from build123d import *

# Parameters (mm, degrees)
SKETCH1_R           = 13.25
SKETCH1_R_2         = 11.25
BOSS_EXTRUDE1_DEPTH = 7
SKETCH2_R           = 20
BOSS_EXTRUDE2_DEPTH = 2
FILLET1_R           = 6
SKETCH3_R           = 11.25
CUT_EXTRUDE1_DEPTH  = 2
FILLET2_R           = 1


with BuildPart() as part:
    # Sketch1 → Boss-Extrude1 (new body)
    with BuildSketch(Plane.XY):
        Circle(SKETCH1_R)
        Circle(SKETCH1_R_2, mode=Mode.SUBTRACT)
    extrude(amount=BOSS_EXTRUDE1_DEPTH)

    # Sketch2 → Boss-Extrude2 (add)
    with BuildSketch(Plane.XY.offset(7)):
        Circle(SKETCH2_R)
    extrude(amount=-BOSS_EXTRUDE2_DEPTH)

    # Fillet1
    # the kernel refuses this fillet: 6 mm, written as the material it adds along each edge
    with BuildSketch(Plane(origin=(0, 0, 5), x_dir=(1, 0, 0), z_dir=(0, 1, 0))) as fillet1_piece_1:
        with BuildLine():
            CenterArc((19.166079783, 6), FILLET1_R, 189.594068227, 80.405931773)
            Line((19.166079783, 0), (19.166079783, -0.12))
            Line((19.166079783, -0.12), (13.25, -0.12))
            Line((13.25, -0.12), (13.13, 0))
            ThreePointArc((13.13, 0), (13.13, 2.5), (13.131678404, 4.98))
            Line((13.131678404, 4.98), (13.25, 5))
        make_face()
    revolve(axis=Axis((0, 0, 5), (0, 0, -1)))

    # Sketch3 → Cut-Extrude1 (cut)
    with BuildSketch(Plane(origin=(0, 0, 5), x_dir=(-1, 0, 0), z_dir=(0, 0, -1))):
        Circle(SKETCH3_R)
    extrude(amount=-CUT_EXTRUDE1_DEPTH, mode=Mode.SUBTRACT)

    # Fillet2
    fillet2_edges = [part.edges().sort_by_distance(p)[0] for p in [
        (-20, 0, 5),
    ]]
    fillet(fillet2_edges, radius=FILLET2_R)


solid = part.part
Input: part model. Units: mm. Frame: model coordinates. Round coordinates to 2 decimals unless told otherwise and drop trailing zeros. Write each loop counter-clockwise with the first axis right and the second up, starting at its lowest first coordinate (ties: lowest second). Pieces come first, ordered by that corner, then holes.
1) Cut plane A-A (z = 1.5). Return the cut outline in (x, y), then the cut area to 3 significant figures.
2) Contact query for flat-ended pins moving along their axis: P1, Ø1, axis at x = -7, z = 1, coming from the +Y side; P2, Ø3, axis at y = 12, z = 2.5, coming from the -X side; P3, Ø4, axis at x = 3, z = 4.5, coming from the -Y side. Output: stop coordinate, or through.
3) Ray query, L1, parallel to Y at x = 0, z = 5.85; L2, parallel to Y at x = 10, z = 1.25; L3, parallel to X at y = 0, z = 3.35. Return the intervals inside material, ascending.
Geometry says:
1. outline: circle Ø27.42 at (0, 0); hole circle Ø22.5 at (0, 0)
1. area: 193 mm2
2. P1: stops at y = 11.92
2. P2: stops at x = -10.76
2. P3: stops at y = -19.93
3. L1: y = -19.99 to -11.25, 11.25 to 19.99
3. L2: y = -9.22 to -5.15, 5.15 to 9.22
3. L3: x = -15.03 to -11.25, 11.25 to 15.03
